The listing builds one solid part. Answer for the finished solid, in the listing's coordinates (mm). Round coordinates to 2 decimals unless told otherwise and drop trailing zeros. Order: outer loops, then holes, each group sorted by start corner. A loop starts at its lowest first (then second) coordinate and runs counter-clockwise, first axis right, second up. Notation, with made-up numbers: (51, 27) - (55, 27) arc R28 cw to (55, 56) - close; hole circle Ø11 at (36.25, 51.5). An arc over 180 degrees is marked (long way). Write item = value, one per line.
Autodesk Inventor part; units mm, degrees
ref_plane "YZ Plane" through (0, 0, 0) normal (1, 0, 0) x (0, 1, 0)
ref_plane "XZ Plane" through (0, 0, 0) normal (0, 1, 0) x (-1, 0, 0)
ref_plane "XY Plane" through (0, 0, 0) normal (0, 0, 1) x (1, 0, 0)
sketch "Sketch1" plane through (0, 0, 0) normal (0, 0, 1) x (1, 0, 0)
  line L0 (-97, 107) -> (97, 107)
  line L1 (97, 107) -> (97, -107)
  line L2 (97, -107) -> (-97, -107)
  line L3 (-97, -107) -> (-97, 107)
  line L4 (-97, 107) -> (97, -107) construction
  line L5 (97, 107) -> (-97, -107) construction
  point P0 (0, 0)
  dimension "d0" = 194
  dimension "d1" = 214
extrude "Plate1" add sketch "Sketch1" along normal blind 4
sketch "Sketch2" plane through (0, 0, 0) normal (0, 0, 1) x (1, 0, 0)
  circle A0 centre (0, 0) radius 45
  dimension "d3" = 90
extrude "Extrusion1" cut sketch "Sketch2" along normal blind 10
equation "\"d2\" = Thickness"
equation "\"BendRadius\" = Thickness"
equation "\"BendReliefWidth\" = Thickness"
equation "\"BendReliefDepth\" = 0.5 * Thickness"
equation "\"CornerReliefSize\" = 4 * Thickness"
equation "\"MinimumRemnant\" = 2 * Thickness"
equation "\"TransitionRadius\" = BendRadius"
equation "\"JacobiRadiusSize\" = BendRadius"
equation "\"GapSize\" = Thickness"
equation "\"Конус_Угол_продольный\" = 52.4deg"
equation "\"Конус_Угол_поперечный\" = 52deg"
properties part number "MSC 111 CONE IN BOTTOM" material "Stainless Steel"
Q1. A flat-ended cylindrical pin translates along its axis: P1, Ø10, axis at x = -75, y = 12.5, coming from the -Z side. Find the tip coordinate at first contact, or state that the pin passes through.
Model answer:
P1 = 0
Q2. Section A-A on y = 0 is taken. Determine the outline of the cut face in (x, z).
Model answer:
outline = (-97, 0) - (-45, 0) - (-45, 4) - (-97, 4) - close; (45, 0) - (97, 0) - (97, 4) - (45, 4) - close
Q3. Section B-B on x = 0 is taken. Determine the outline of the cut face in (y, z).
Model answer:
outline = (-107, 0) - (-45, 0) - (-45, 4) - (-107, 4) - close; (45, 0) - (107, 0) - (107, 4) - (45, 4) - close
Q4. Section C-C on z = 1.3 is taken. Determine the outline of the cut face in (x, y), then the cut area to 3 significant figures.
Model answer:
outline = (-97, -107) - (97, -107) - (97, 107) - (-97, 107) - close; hole circle Ø90 at (0, 0)
area = 35,200 mm^2
Q5. Find the intervals of material crossed by line 1 (Y direction, x = 0, z = 2.75); line 2 (X direction, y = 0, z = 1.95); line 3 (Y direction, x = 8, z = 0.3), in increasing order. Write a range as from..to.
Model answer:
line_1 = -107..-45, 45..107
line_2 = -97..-45, 45..97
line_3 = -107..-44.28, 44.28..107
Q6. Determine the mould class of faces 1 (the face through (20.765, 39.923, 1.972)), 2 (the face through (-1, -46, 0)) for opening direction Y: released by +Y, released by -Y, zero draft, split by the parting line, or undercut.
Model answer:
face_1 = undercut
face_2 = zero draft
